Check sheet for the modelled part. Datum: model origin and axes. Units: mm. A direction names the side the tool comes from. Round coordinates to 2 decimals unless told otherwise and drop trailing zeros. Loops run counter-clockwise (first coordinate to the right, second up) from the corner with the lowest first, then second, coordinate; pieces in that order, holes last. Notation, with made-up numbers: (42, 83) - (98, 83) arc R20 ccw to (98, 101) - close; hole circle Ø3 at (84.25, 5). An arc over 180 degrees is marked (long way). Put each result on its own line as item: value. Start each with the question number.
Item 1: Tool access check on faces 1 (the cylindrical face through (-8.845, -40.49, -0.921)), 2 (the cylindrical face through (4.88, 0.49, -1.08)), 3 (the flat face through (0, -15, -40)). Record the directions out of +Z, -Z, +X, -X, +Y, -Y that give a thin tool (end or side, any length) a straight path to the whole face; none if there is none.
Item 2: Gauge pin test, flat ends, axial feed: pin 1 Ø8 at (x, z) = (0, 0) entering from -Y; pin 2 Ø3 at (x, y) = (8.5, -33) entering from +Z; pin 3 Ø10 at (y, z) = (-22.5, -37) entering from -X; pin 4 Ø3.5 at (x, z) = (10, -100) entering from +Y. Record the tip position at first contact, or that the pin passes through.
Item 3: Draft check along Y on faces 4 (the flat face through (0, 0, -10)), 5 (the flat face through (0, -1.5, -5)), 6 (the flat face through (5, -35, -105)). Enter one of: pulls with the +Y half, pulls with the -Y half, needs draft (parallel to the pull), parting line crosses it, or undercut.
Item 4: Material ranges on line 1 along Y through (x, z) = (-7.5, -19); line 2 along Y through (x, z) = (-1, -56.5); line 3 along Z through (x, y) = (0.25, -13.5), recorded low to high.
Item 5: Section check A-A, the plane z = -8. Record the cut outline in (x, y), and give its area (3 significant figures).
Item 6: Section check B-B, the plane y = -12. Record the cut outline in (x, z).
Item 7: Section check C-C, the plane z = -55. Record the cut outline in (x, y), and give its area (3 significant figures).
from build123d import *

# Parameters (mm, degrees)
SKETCH3_R           = 4.249999999999999
SKETCH3_R_2         = 2.1999999999999984
BOSS_EXTRUDE2_DEPTH = 1.5
SKETCH3_18_R        = 5
SKETCH3_18_R_2      = 1.5
BOSS_EXTRUDE3_DEPTH = 1
SKETCH3_19_R        = 4.249999999999999
SKETCH3_19_R_2      = 3.250000000000001
BOSS_EXTRUDE4_DEPTH = 2.5
BOSS_EXTRUDE5_START = 39.75
SKETCH3_20_R        = 5
SKETCH3_20_R_2      = 1.2500000000000002
SKETCH3_20_R_3      = 1.2499999999999998
SKETCH3_20_R_4      = 1.2499999999999991
SKETCH3_20_R_5      = 1.2500000000000004
SKETCH3_20_R_6      = 2.1999999999999984
BOSS_EXTRUDE5_DEPTH = 1.5
SKETCH3_21_R        = 2.1999999999999984
BOSS_EXTRUDE6_DEPTH = 41.25
SKETCH3_23_R        = 2.1999999999999984
CUT_EXTRUDE7_DEPTH  = 30.63
CUT_EXTRUDE8_START  = 38.63
SKETCH3_24_R        = 2.1999999999999984
CUT_EXTRUDE8_DEPTH  = 2.62
FILLET5_R           = 10
FILLET6_R           = 10
FILLET7_R           = 2


with BuildPart() as part:
    # Sketch3 → Boss-Extrude2 (new body)
    with BuildSketch(Plane(origin=(0, 0, 0), x_dir=(-1, 0, 0), z_dir=(0, -1, 0))):
        with BuildLine():
            Line((5.000000000000005, 100), (10.980122362164348, 0.6609938818917814))
            ThreePointArc((10.980122362164348, 0.6609938818917814), (0.3306463489834291, -10.995029467532314), (-11, 0))
            Line((-11, 0), (-5.300000000000002, 95.00000000000001))
            Line((-5.300000000000002, 95.00000000000001), (-9.999999999999998, 95.00000000000003))
            ThreePointArc((-9.999999999999998, 95.00000000000003), (-15.00000000000001, 100.00000000000003), (-9.999999999999996, 105.00000000000004))
            Line((-9.999999999999996, 105.00000000000004), (5.6e-16, 105.00000000000003))
            ThreePointArc((5.6e-16, 105.00000000000003), (3.5355339059327497, 103.53553390593275), (5.000000000000005, 100))
        make_face()
        with Locations(Location((0, 0, 0), (0, 0, 270))):
            Circle(SKETCH3_R, mode=Mode.SUBTRACT)
        with Locations(Location((-9.999999999999998, 100.00000000000003, 0), (0, 0, 270))):
            Circle(SKETCH3_R_2, mode=Mode.SUBTRACT)
    extrude(amount=BOSS_EXTRUDE2_DEPTH)

    # Sketch3<18> → Boss-Extrude3 (add)
    with BuildSketch(Plane(origin=(0, 0, 0), x_dir=(-1, 0, 0), z_dir=(0, -1, 0))):
        with Locations(Location((0, 0, 0), (0, 0, 270))):
            Circle(SKETCH3_18_R)
        with Locations(Location((0, 0, 0), (0, 0, 270))):
            Circle(SKETCH3_18_R_2, mode=Mode.SUBTRACT)
    extrude(amount=-BOSS_EXTRUDE3_DEPTH)

    # Sketch3<19> → Boss-Extrude4 (add)
    with BuildSketch(Plane(origin=(0, 0, 0), x_dir=(-1, 0, 0), z_dir=(0, -1, 0))):
        with Locations(Location((0, 0, 0), (0, 0, 270))):
            Circle(SKETCH3_19_R)
        with Locations(Location((0, 0, 0), (0, 0, 270))):
            Circle(SKETCH3_19_R_2, mode=Mode.SUBTRACT)
    extrude(amount=BOSS_EXTRUDE4_DEPTH)



with BuildPart() as body_2:
    # Sketch3<20> → Boss-Extrude5 (new body)
    with BuildSketch(Plane(origin=(0, 0, 0), x_dir=(-1, 0, 0), z_dir=(0, -1, 0)).offset(BOSS_EXTRUDE5_START)):
        with BuildLine():
            Line((5.000000000000005, 100), (10.980122362164348, 0.6609938818917814))
            ThreePointArc((10.980122362164348, 0.6609938818917814), (0.3306463489834291, -10.995029467532314), (-11, 0))
            Line((-11, 0), (-5.300000000000002, 95.00000000000001))
            Line((-5.300000000000002, 95.00000000000001), (-9.999999999999998, 95.00000000000003))
            ThreePointArc((-9.999999999999998, 95.00000000000003), (-15.00000000000001, 100.00000000000003), (-9.999999999999996, 105.00000000000004))
            Line((-9.999999999999996, 105.00000000000004), (5.6e-16, 105.00000000000003))
            ThreePointArc((5.6e-16, 105.00000000000003), (3.5355339059327497, 103.53553390593275), (5.000000000000005, 100))
        make_face()
        with Locations(Location((0, 0, 0), (0, 0, 270))):
            Circle(SKETCH3_20_R, mode=Mode.SUBTRACT)
        with Locations(Location((-8, 0, 0), (0, 0, 270))):
            Circle(SKETCH3_20_R_2, mode=Mode.SUBTRACT)
        with Locations(Location((-5.65685424949238, 5.656854249492384, 0), (0, 0, 270))):
            Circle(SKETCH3_20_R_2, mode=Mode.SUBTRACT)
        with Locations(Location((0, 8.000000000000007, 0), (0, 0, 270))):
            Circle(SKETCH3_20_R_3, mode=Mode.SUBTRACT)
        with Locations(Location((5.656854249492385, 5.656854249492391, 0), (0, 0, 270))):
            Circle(SKETCH3_20_R_2, mode=Mode.SUBTRACT)
        with Locations(Location((8.000000000000009, 9.11e-15, 0), (0, 0, 270))):
            Circle(SKETCH3_20_R_4, mode=Mode.SUBTRACT)
        with Locations(Location((5.656854249492392, -5.656854249492377, 0), (0, 0, 270))):
            Circle(SKETCH3_20_R_2, mode=Mode.SUBTRACT)
        with Locations(Location((1.019e-14, -8, 0), (0, 0, 270))):
            Circle(SKETCH3_20_R_5, mode=Mode.SUBTRACT)
        with Locations(Location((-5.656854249492376, -5.656854249492382, 0), (0, 0, 270))):
            Circle(SKETCH3_20_R_2, mode=Mode.SUBTRACT)
        with Locations(Location((-9.999999999999998, 100.00000000000003, 0), (0, 0, 270))):
            Circle(SKETCH3_20_R_6, mode=Mode.SUBTRACT)
    extrude(amount=BOSS_EXTRUDE5_DEPTH)


with BuildPart() as part_1:
    add(part.part)

    add(body_2.part)  # Boss-Extrude6 merges body 2
    # Sketch3<21> → Boss-Extrude6 (add)
    with BuildSketch(Plane(origin=(0, 0, 0), x_dir=(-1, 0, 0), z_dir=(0, -1, 0))):
        with BuildLine():
            ThreePointArc((5.000000000000007, 100), (3.5355339059327426, 103.53553390593274), (6e-17, 105))
            Line((0, 105.00000000000003), (-9.999999999999996, 105.00000000000004))
            ThreePointArc((-9.999999999999996, 105.00000000000003), (-15.000000000000014, 100.00000000000003), (-9.999999999999998, 95.00000000000003))
            Line((-9.999999999999998, 95.00000000000003), (-5.300000000000002, 95.00000000000001))
            Line((-5.300000000000002, 95.00000000000001), (-9.800000000000002, 20))
            ThreePointArc((-9.800000000000002, 20), (0.00796544916277364, 22.5700311604401), (9.815930898325552, 19.999999999999996))
            Line((9.815930898325552, 19.999999999999996), (5.000000000000004, 100))
        make_face()
        with Locations(Location((-9.999999999999998, 100.00000000000003, 0), (0, 0, 270))):
            Circle(SKETCH3_21_R, mode=Mode.SUBTRACT)
    extrude(amount=BOSS_EXTRUDE6_DEPTH)

    # Sketch3<23> → Cut-Extrude7 (cut)
    with BuildSketch(Plane(origin=(0, 0, 0), x_dir=(-1, 0, 0), z_dir=(0, -1, 0))):
        with BuildLine():
            Line((8.611948173744162, 40), (5.000000000000005, 100))
            ThreePointArc((5.000000000000002, 100), (3.5355339059327484, 103.53553390593275), (5.6e-16, 105.00000000000003))
            Line((0, 105.00000000000003), (-9.999999999999996, 105.00000000000004))
            ThreePointArc((-9.999999999999996, 105.00000000000003), (-15.000000000000014, 100.00000000000003), (-9.999999999999998, 95.00000000000003))
            Line((-9.999999999999998, 95.00000000000003), (-5.300000000000002, 95.00000000000001))
            Line((-5.300000000000002, 95.00000000000001), (-8.600000000000001, 40.00000000000001))
            Line((-8.600000000000003, 40), (8.611948173744162, 40))
        make_face()
        with Locations(Location((-9.999999999999998, 100.00000000000003, 0), (0, 0, 270))):
            Circle(SKETCH3_23_R, mode=Mode.SUBTRACT)
    extrude(amount=CUT_EXTRUDE7_DEPTH, mode=Mode.SUBTRACT)

    # Sketch3<24> → Cut-Extrude8 (cut)
    with BuildSketch(Plane(origin=(0, 0, 0), x_dir=(-1, 0, 0), z_dir=(0, -1, 0)).offset(CUT_EXTRUDE8_START)):
        with BuildLine():
            Line((8.611948173744162, 40), (5.000000000000005, 100))
            ThreePointArc((5.000000000000002, 100), (3.5355339059327484, 103.53553390593275), (5.6e-16, 105.00000000000003))
            Line((0, 105.00000000000003), (-9.999999999999996, 105.00000000000004))
            ThreePointArc((-9.999999999999996, 105.00000000000003), (-15.000000000000014, 100.00000000000003), (-9.999999999999998, 95.00000000000003))
            Line((-9.999999999999998, 95.00000000000003), (-5.300000000000002, 95.00000000000001))
            Line((-5.300000000000002, 95.00000000000001), (-8.600000000000001, 40.00000000000001))
            Line((-8.600000000000003, 40), (8.611948173744162, 40))
        make_face()
        with Locations(Location((-9.999999999999998, 100.00000000000003, 0), (0, 0, 270))):
            Circle(SKETCH3_24_R, mode=Mode.SUBTRACT)
    extrude(amount=CUT_EXTRUDE8_DEPTH, mode=Mode.SUBTRACT)

    # Fillet5
    # the kernel refuses this fillet: 10 mm, written as the material it takes off along each edge
    with BuildSketch(Plane(origin=(33.6, 0, -40), x_dir=(0, -1, 0), z_dir=(-1, 0, 0))) as fillet5_piece_1:
        with BuildLine():
            CenterArc((FILLET5_R, FILLET5_R), FILLET5_R, 180, 90)
            Line((-1.78e-15, FILLET5_R), (-FILLET5_R * 0.02, FILLET5_R))
            Line((-FILLET5_R * 0.02, FILLET5_R), (-FILLET5_R * 0.02, -FILLET5_R * 0.02))
            Line((-FILLET5_R * 0.02, -FILLET5_R * 0.02), (FILLET5_R, -FILLET5_R * 0.02))
            Line((FILLET5_R, -FILLET5_R * 0.02), (FILLET5_R, 0))
        make_face()
    extrude(amount=67.21194817374416, mode=Mode.SUBTRACT)
    with BuildSketch(Plane(origin=(25.470017783037456, -41.25, -40), x_dir=(0, 1, 0), z_dir=(-1, 0, 0))) as fillet5_piece_2:
        with BuildLine():
            CenterArc((10, -6.748007113214982), FILLET5_R, 137.5613237933639, 42.4386762066361)
            Line((0, -6.748007113214982), (-0.20000000000000284, -6.748007113214982))
            Line((-0.20000000000000284, -6.748007113214982), (-0.20000000000000284, 0))
            Line((-0.20000000000000284, 0), (0, 0.20000000000000284))
            ThreePointArc((0, 0.20000000000000284), (1.3100000000000023, 0.20000000000000284), (2.4724000000000004, 0.13496014226429764))
            Line((2.4724000000000004, 0.13496014226429764), (2.6199999999999974, 0))
        make_face()
    extrude(amount=50.95198373981907, mode=Mode.SUBTRACT)

    # Fillet6
    fillet6_edges = [part_1.edges().sort_by_distance(p)[0] for p in [
        (-0.00597408687207945, -30.63, -40),
        (-0.00597408687207945, -38.63, -40),
    ]]
    fillet(fillet6_edges, radius=FILLET6_R)

    # Fillet7
    fillet7_edges = [part_1.edges().sort_by_distance(p)[0] for p in [
        (5.300000000000002, -34.63, -95.00000000000001),
        (-0.00796544916277897, -1.5, -22.570031160440095),
        (-0.00796544916277897, -39.75, -22.570031160440095),
    ]]
    fillet(fillet7_edges, radius=FILLET7_R)


solid = part_1.part
Check result:
1. face 1: -Y
1. face 2: +Y
1. face 3: -Z, +X, -X, +Y
2. pin 1: y = -2.5
2. pin 2: z = -20
2. pin 3: x = -9.09
2. pin 4: through
3. face 4: pulls with the +Y half
3. face 5: undercut
3. face 6: needs draft
4. line 1: -41.25 to -39.75, -1.5 to 0
4. line 2: -38.63 to -30.63
4. line 3: -40 to -22.57
5. outline: (-10.54, -41.25) - (-1.25, -41.25) - (-1.25, -39.75) - (-10.54, -39.75) - close; (-10.54, -1.5) - (10.52, -1.5) - (10.52, 0) - (-10.54, 0) - close; (1.25, -41.25) - (10.52, -41.25) - (10.52, -39.75) - (1.25, -39.75) - close
5. area: 59.4 mm²
6. outline: (-9.82, -20) - (-8.61, -40) - (8.6, -40) - (9.8, -20) arc R20 cw to start
7. outline: (-7.71, -38.63) - (7.7, -38.63) - (7.7, -30.63) - (-7.71, -30.63) - close
7. area: 123 mm²
